Source: CAD feature listing. Evaluate the final solid. Frame: model axes, mm. A direction names the side the tool comes from. Coordinates: 2 decimals unless noted, no trailing zeros.
Item 1: Mould query, pull axis Y, two halves, no side actions, for faces 3 (the flat face through (-2, -9, 1.5)), 4 (the cylindrical face through (0.273, -12.918, 0.74)). Classes: released by +Y, released by -Y, zero draft, split by the parting line, or undercut.
Item 2: Ray query, line 1 (Y direction, x = -85, z = 0.55); line 2 (Y direction, x = -50.5, z = 0.95); line 3 (Y direction, x = -55.5, z = 1.2). Return the intervals inside material, ascending.
Item 3: Contact query for a flat-ended pin moving along its axis: P1, Ø3, axis at x = -55, y = 15, coming from the +Z side. Output: stop coordinate, or through.
Item 4: Reachability of faces 1 (the flat face through (17.101, -0.402, 0.74)), 2 (the flat face through (-2, -9, 0)) from +Z, -Z, +X, -X, +Y, -Y: full face, straight path, thin tool, end or side. Return the list, or none.
Item 5: Section A-A on z = 0.5. State how many separate pieces and enclosed holes the cut face has, then the cut area to 3 significant figures.
from build123d import *

# Parameters (mm, degrees)
SKETCH_1_W          = 225
SKETCH_1_H          = 40
EXTRUDE_1_DEPTH     = 1.5
SKETCH_2_R          = 11
SKETCH_2_R_2        = 2.1
CUT_EXTRUDE_1_DEPTH = 115.273794021
SKETCH_3_R          = 11
SKETCH_3_R_2        = 2.1
SKETCH_3_R_3        = 1.7
CUT_EXTRUDE_2_DEPTH = 115.273794021


with BuildPart() as part:
    # 草图1 → 凸台-拉伸1 (new body)
    with BuildSketch(Plane.XY):
        Rectangle(SKETCH_1_W, SKETCH_1_H)
    extrude(amount=EXTRUDE_1_DEPTH)

    # 草图2 → 切除-拉伸1 (cut, through all)
    with BuildSketch(Plane(origin=(0, 0, 0), x_dir=(-1, 0, 0), z_dir=(0, 0, -1))):
        with Locations((85, 0)):
            Circle(SKETCH_2_R)
        with Locations((55, 0)):
            Circle(SKETCH_2_R)
        with Locations((30, 15)):
            Circle(SKETCH_2_R_2)
        with Locations((0, -15)):
            Circle(SKETCH_2_R_2)
        with Locations((-30, 15)):
            Circle(SKETCH_2_R_2)
        with Locations((-85, 0)):
            Circle(SKETCH_2_R)
        with Locations((-55, 0)):
            Circle(SKETCH_2_R)
        with BuildLine():
            Line((-6.826276619, -7.251924558), (-27.667949706, 6.642524166))
            ThreePointArc((-27.667949706, 6.642524166), (-29.207786888, 6.716960623), (-30, 5.394448725))
            Line((-30, 5.394448725), (-30, -8.5))
            ThreePointArc((-30, -8.5), (-29.560660172, -9.560660172), (-28.5, -10))
            Line((-28.5, -10), (-7.658326913, -10))
            ThreePointArc((-7.658326913, -10), (-6.222688873, -8.934676223), (-6.826276619, -7.251924558))
        make_face()
        with BuildLine():
            Line((-1.5, -4.394448725), (-1.5, 8.5))
            ThreePointArc((-1.5, 8.5), (-1.939339828, 9.560660172), (-3, 10))
            Line((-3, 10), (-22.341673087, 10))
            ThreePointArc((-22.341673087, 10), (-23.777311127, 8.934676223), (-23.173723381, 7.251924558))
            Line((-23.173723381, 7.251924558), (-3.832050294, -5.642524166))
            ThreePointArc((-3.832050294, -5.642524166), (-2.292213112, -5.716960623), (-1.5, -4.394448725))
        make_face()
        with BuildLine():
            Line((3.832050294, -5.642524166), (23.173723381, 7.251924558))
            ThreePointArc((23.173723381, 7.251924558), (23.777311127, 8.934676223), (22.341673087, 10))
            Line((22.341673087, 10), (3, 10))
            ThreePointArc((3, 10), (1.939339828, 9.560660172), (1.5, 8.5))
            Line((1.5, 8.5), (1.5, -4.394448725))
            ThreePointArc((1.5, -4.394448725), (2.292213112, -5.716960623), (3.832050294, -5.642524166))
        make_face()
        with BuildLine():
            Line((30, -8.5), (30, 5.394448725))
            ThreePointArc((30, 5.394448725), (29.207786888, 6.716960623), (27.667949706, 6.642524166))
            Line((27.667949706, 6.642524166), (6.826276619, -7.251924558))
            ThreePointArc((6.826276619, -7.251924558), (6.222688873, -8.934676223), (7.658326913, -10))
            Line((7.658326913, -10), (28.5, -10))
            ThreePointArc((28.5, -10), (29.560660172, -9.560660172), (30, -8.5))
        make_face()
    extrude(amount=-CUT_EXTRUDE_1_DEPTH, mode=Mode.SUBTRACT)

    # 草图3 → 切除-拉伸2 (cut, through all)
    with BuildSketch(Plane(origin=(0, 0, 0), x_dir=(-1, 0, 0), z_dir=(0, 0, -1))):
        with Locations((85, 0)):
            Circle(SKETCH_3_R)
        with Locations((55, 0)):
            Circle(SKETCH_3_R)
        with Locations((0, -15)):
            Circle(SKETCH_3_R_2)
        with Locations((-55, 0)):
            Circle(SKETCH_3_R)
        with Locations((30, 15)):
            Circle(SKETCH_3_R_2)
        with Locations((-30, 15)):
            Circle(SKETCH_3_R_2)
        with Locations((-85, 0)):
            Circle(SKETCH_3_R)
        with Locations((55, -15)):
            Circle(SKETCH_3_R_3)
        with Locations((85, -15)):
            Circle(SKETCH_3_R_3)
        with Locations((-37, 0)):
            Circle(SKETCH_3_R_3)
        with Locations((37, 0)):
            Circle(SKETCH_3_R_3)
        with Locations((70, 0)):
            Circle(SKETCH_3_R_3)
        with Locations((-109.5, 0)):
            Circle(SKETCH_3_R_3)
        with Locations((-85, -15)):
            Circle(SKETCH_3_R_3)
        with Locations((109.5, 0)):
            Circle(SKETCH_3_R_3)
        with Locations((-70, 0)):
            Circle(SKETCH_3_R_3)
        with Locations((-55, 15)):
            Circle(SKETCH_3_R_3)
        with Locations((85, 15)):
            Circle(SKETCH_3_R_3)
        with Locations((-85, 15)):
            Circle(SKETCH_3_R_3)
        with Locations((-55, -15)):
            Circle(SKETCH_3_R_3)
        with Locations((55, 15)):
            Circle(SKETCH_3_R_3)
        with BuildLine():
            Line((-23.173723381, 7.251924558), (-3.832050294, -5.642524166))
            ThreePointArc((-3.832050294, -5.642524166), (-2.292213112, -5.716960623), (-1.5, -4.394448725))
            Line((-1.5, -4.394448725), (-1.5, 8.5))
            ThreePointArc((-1.5, 8.5), (-1.939339828, 9.560660172), (-3, 10))
            Line((-3, 10), (-22.341673087, 10))
            ThreePointArc((-22.341673087, 10), (-23.777311127, 8.934676223), (-23.173723381, 7.251924558))
        make_face()
        with BuildLine():
            Line((-30, 5.394448725), (-30, -8.5))
            ThreePointArc((-30, -8.5), (-29.560660172, -9.560660172), (-28.5, -10))
            Line((-28.5, -10), (-7.658326913, -10))
            ThreePointArc((-7.658326913, -10), (-6.222688873, -8.934676223), (-6.826276619, -7.251924558))
            Line((-6.826276619, -7.251924558), (-27.667949706, 6.642524166))
            ThreePointArc((-27.667949706, 6.642524166), (-29.207786888, 6.716960623), (-30, 5.394448725))
        make_face()
        with BuildLine():
            Line((27.667949706, 6.642524166), (6.826276619, -7.251924558))
            ThreePointArc((6.826276619, -7.251924558), (6.222688873, -8.934676223), (7.658326913, -10))
            Line((7.658326913, -10), (28.5, -10))
            ThreePointArc((28.5, -10), (29.560660172, -9.560660172), (30, -8.5))
            Line((30, -8.5), (30, 5.394448725))
            ThreePointArc((30, 5.394448725), (29.207786888, 6.716960623), (27.667949706, 6.642524166))
        make_face()
        with BuildLine():
            Line((1.5, 8.5), (1.5, -4.394448725))
            ThreePointArc((1.5, -4.394448725), (2.292213112, -5.716960623), (3.832050294, -5.642524166))
            Line((3.832050294, -5.642524166), (23.173723381, 7.251924558))
            ThreePointArc((23.173723381, 7.251924558), (23.777311127, 8.934676223), (22.341673087, 10))
            Line((22.341673087, 10), (3, 10))
            ThreePointArc((3, 10), (1.939339828, 9.560660172), (1.5, 8.5))
        make_face()
    extrude(amount=-CUT_EXTRUDE_2_DEPTH, mode=Mode.SUBTRACT)


solid = part.part
Answer list:
1. face 3: zero draft
1. face 4: undercut
2. line 1: y = -20 to -16.7, -13.3 to -11, 11 to 13.3, 16.7 to 20
2. line 2: y = -20 to -10.04, 10.04 to 20
2. line 3: y = -20 to -16.62, -13.38 to -10.99, 10.99 to 13.38, 16.62 to 20
3. P1: passes through
4. face 1: +Z, -Z
4. face 2: -Z, +X, -X, +Y, -Y
5. separate pieces: 1
5. enclosed holes: 25
5. area: 6,400 mm2
